```python
from build123d import *

# Parameters (mm, degrees)
F0_W     = 150
F0_H     = 158
F1_DEPTH = 15
F2_R     = 50
F2_R_2   = 45
F3_DEPTH = 250
F4_R     = 5
F4_R_2   = 3.5
F5_DEPTH = 250
F6_R     = 10
F7_R     = 10
F8_DEPTH = 100


with BuildPart() as f1:
    # F0 (on Front) → F1 (new body)
    with BuildSketch(Plane.XZ):
        Rectangle(F0_W, F0_H)
    extrude(amount=F1_DEPTH)

    # F2 (on Front) → F3 (join)
    with BuildSketch(Plane.XZ):
        Circle(F2_R)
        Circle(F2_R_2, mode=Mode.SUBTRACT)
    extrude(amount=-F3_DEPTH)

    # F4 (on Front) → F5 (join)
    with BuildSketch(Plane.XZ):
        with Locations((60, 0)):
            Circle(F4_R)
        with Locations((60, 0)):
            Circle(F4_R_2, mode=Mode.SUBTRACT)
    extrude(amount=-F5_DEPTH)

    # F6
    f6_edges = [f1.edges().sort_by_distance(p)[0] for p in [
        (75, -7.5, 79),
        (-75, -7.5, 79),
        (-75, -7.5, -79),
        (75, -7.5, -79),
    ]]
    fillet(f6_edges, radius=F6_R)

    # F7 (on Front) → F8 (join)
    with BuildSketch(Plane.XZ):
        with Locations((60, 0)):
            Circle(F7_R)
    extrude(amount=F8_DEPTH)


solid = f1.part
```
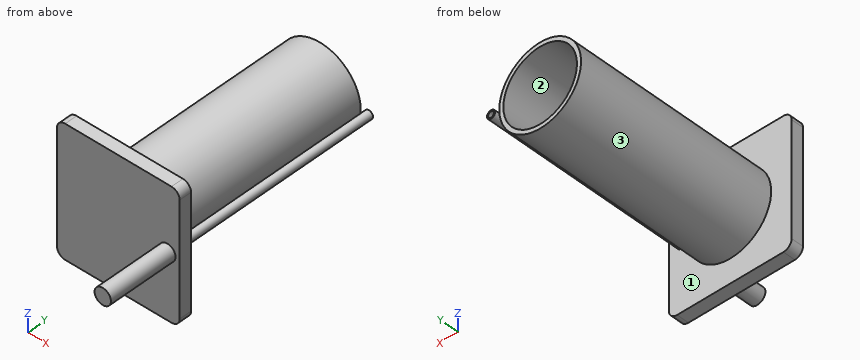
Geometry check sheet. Reference: the model listing, model coordinates, mm. Face numbers are marked on the shaded views. Coordinates: 2 decimals unless noted, no trailing zeros. Order: outer loops, then holes, each group sorted by start corner. A loop starts at its lowest first (then second) coordinate and runs counter-clockwise, first axis right, second up. Notation, with made-up numbers: M 71,43.5 L 115,43.5 A32 ccw 115,76.5 Z; hole C 22,13.25 d10. An arc over 180 degrees is marked long. Answer as a JSON object with one key per item and string values.
Q1. Cross-section at D-D on y = -52. Record the cut outline in (x, z).
Results are:
{"outline": "C 60,0 d20"}
Q2. Scan lines: line 1 (Z direction, x = 0, y = 90); line 2 (Z direction, x = 60, y = 115); line 3 (Y direction, x = 26.5, z = -59.5). Record each from-to range of solid material in increasing order.
Results are:
{"line 1": "z = -50 to -45, 45 to 50", "line 2": "z = -5 to -3.5, 3.5 to 5", "line 3": "y = -15 to 0"}
Q3. Release check for a two-part mould opening along Z. For the marked faces 1, 2 and 3 record: released by +Z, released by -Z, zero draft, split by the parting line, or undercut.
Results are:
{"face 1": "zero draft", "face 2": "undercut", "face 3": "split by the parting line"}
Q4. Cross-section at C-C on z = 0. Record the cut outline in (x, y), and give its area (3 significant figures).
Results are:
{"outline": "M -75,-15 L 50,-15 L 50,-100 L 70,-100 L 70,-15 L 75,-15 L 75,0 L 65,0 L 65,250 L 63.5,250 L 63.5,0 L 56.5,0 L 56.5,250 L 55,250 L 55,0 L 50,0 L 50,250 L 45,250 L 45,0 L -45,0 L -45,250 L -50,250 L -50,0 L -75,0 Z", "area": "7,200 mm²"}
Q5. Cross-section at B-B on x = 60. Record the cut outline in (y, z).
Results are:
{"outline": "M -100,-10 L -15,-10 L -15,-79 L 0,-79 L 0,-5 L 250,-5 L 250,-3.5 L 0,-3.5 L 0,3.5 L 250,3.5 L 250,5 L 0,5 L 0,79 L -15,79 L -15,10 L -100,10 Z"}
Q6. Depth check by flat-ended pin: pin 1 Ø3.5 at (x, z) = (60, 1.5) entering from +Y; pin 2 Ø3 at (y, z) = (211.5, 38) entering from -X; pin 3 Ø9 at (x, z) = (60, 0) entering from +Y; pin 4 Ø12 at (x, z) = (0, -21) entering from -Y. Enter the tip coordinate at first touch or a pass-through.
Results are:
{"pin 1": "stops at y = 0", "pin 2": "stops at x = -34.17", "pin 3": "stops at y = 250", "pin 4": "stops at y = -15"}
Q7. Cross-section at A-A on y = 4. Record the cut outline in (x, z).
Results are:
{"outline": "C 0,0 d100; C 60,0 d10; hole C 0,0 d90; hole C 60,0 d7"}
